Geometry: see drawing. Coordinates: mm, zero at the bounding-box minimum. A direction names the side the tool comes from. Coordinates: 2 decimals unless noted, no trailing zeros. Loops run counter-clockwise (first coordinate to the right, second up) from the corner with the lowest first, then second, coordinate; pieces in that order, holes last.
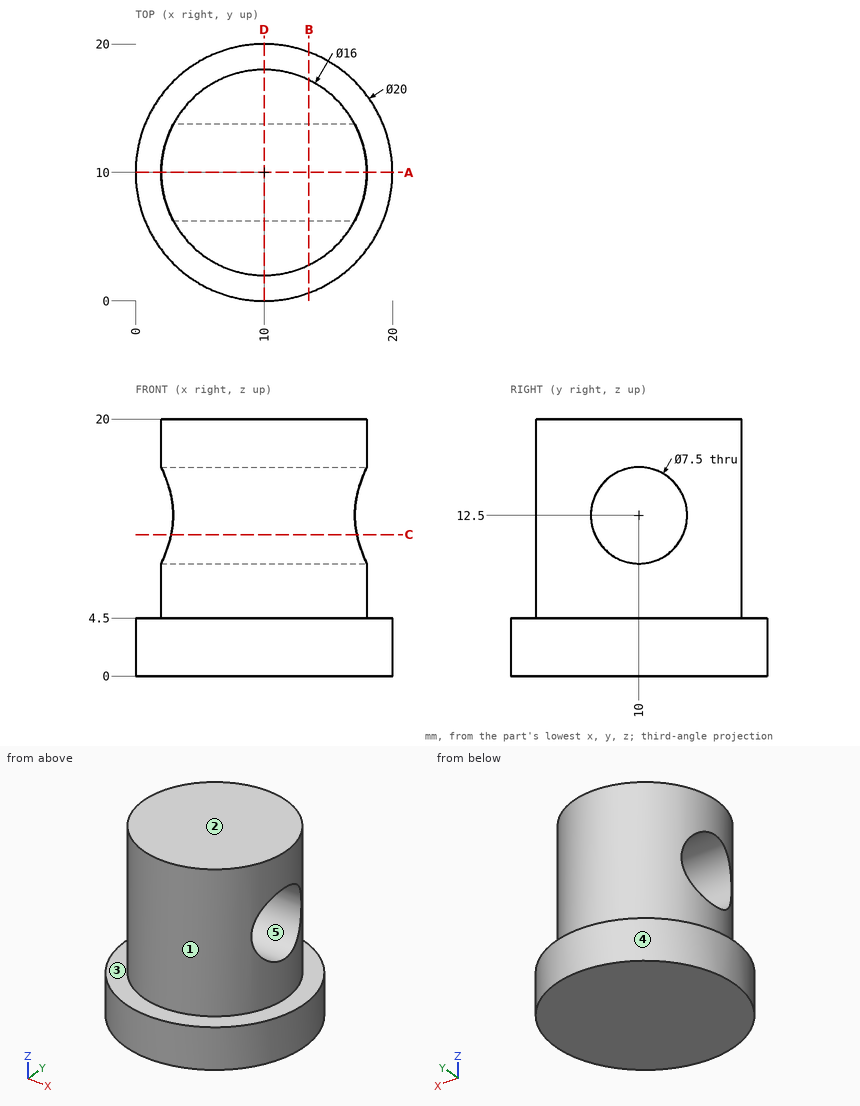
Item 1: Section query D-D (x = 10). Output: boundary loops of the cut face in (y, z).
Result:
outline: (0, 0) - (20, 0) - (20, 4.5) - (18, 4.5) - (18, 20) - (2, 20) - (2, 4.5) - (0, 4.5) - close; hole circle Ø7.5 at (10, 12.5)
Item 2: Mould query, pull axis Y, two halves, no side actions, for the marked faces 3, 4 and 5. Classes: +Y half, -Y half, draft (parallel to the pull), parting line (faces both ways), or undercut.
Result:
face 3: draft
face 4: parting line
face 5: undercut
Item 3: Reachability of the marked faces 1 and 2 from +Z, -Z, +X, -X, +Y, -Y: full face, straight path, thin tool, end or side. Return the list, or none.
Result:
face 1: +Z
face 2: +Z, +X, -X, +Y, -Y
Item 4: Contact query for flat-ended pins moving along their axis: P1, Ø10, axis at y = 14, z = 2.5, coming from the +X side; P2, Ø12, axis at x = 17.5, z = 16.5, coming from the +Y side; P3, Ø1.5, axis at y = 4, z = 12, coming from the -X side; P4, Ø12, axis at x = 17.5, z = 14.5, coming from the -Y side. Output: stop coordinate, or through.
Result:
P1: stops at x = 20
P2: stops at y = 17.86
P3: stops at x = 3.96
P4: stops at y = 2.14
Item 5: Section query B-B (x = 13.5). Output: boundary loops of the cut face in (y, z), then the cut area to 3 significant figures.
Result:
outline: (0.63, 0) - (19.37, 0) - (19.37, 4.5) - (17.19, 4.5) - (17.19, 20) - (2.81, 20) - (2.81, 4.5) - (0.63, 4.5) - close; hole circle Ø7.5 at (10, 12.5)
area: 263 mm2
Item 6: Section query A-A (y = 10). Output: boundary loops of the cut face in (x, z).
Result:
outline: (0, 0) - (20, 0) - (20, 4.5) - (18, 4.5) - (18, 8.75) - (2, 8.75) - (2, 4.5) - (0, 4.5) - close; (2, 16.25) - (18, 16.25) - (18, 20) - (2, 20) - close
Item 7: Section query C-C (z = 11). Output: boundary loops of the cut face in (x, y), then the cut area to 3 significant figures.
Result:
outline: (2.78, 6.56) arc R8 ccw to (17.22, 6.56) - close; (2.78, 13.44) - (17.22, 13.44) arc R8 ccw to start
area: 94.6 mm2
Item 8: Line query: L1, parallel to Z at x = 6.75, y = 10; L2, parallel to Y at x = 10.25, z = 12.5; L3, parallel to Y at x = 7.5, z = 12.5. Output: solid intervals per line, ascending.
Result:
L1: z = 0 to 8.75, 16.25 to 20
L2: y = 2 to 6.25, 13.75 to 18
L3: y = 2.4 to 6.25, 13.75 to 17.6
